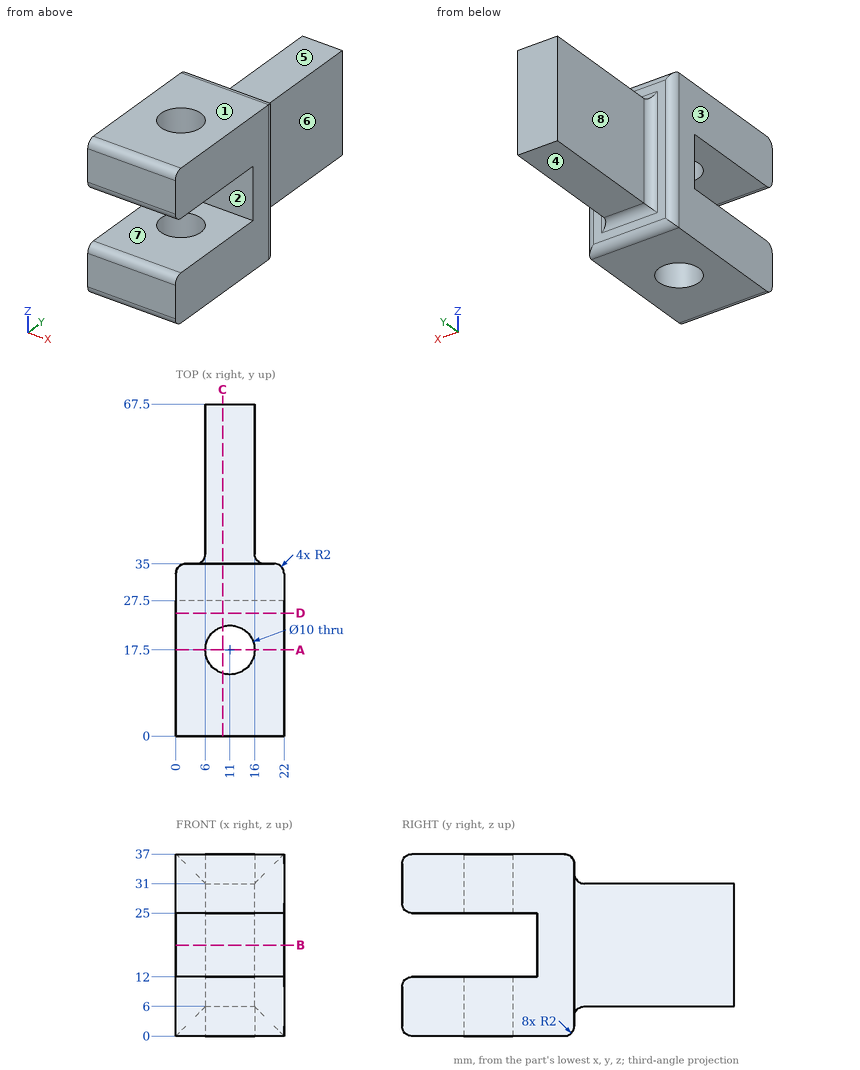
Verification items for this drawing (mm, ordinates from the low corner). A direction names the side the tool comes from. Round coordinates to 2 decimals unless told otherwise and drop trailing zeros. Order: outer loops, then holes, each group sorted by start corner. A loop starts at its lowest first (then second) coordinate and runs counter-clockwise, first axis right, second up. Notation, with made-up numbers: (34.5, 50.25) -> (88.5, 50.25) arc R11 cw to (88.5, 58.25) -> close; hole circle Ø1 at (40.5, -39). An arc over 180 degrees is marked (long way). Use one line per item in the form item = value.
1. Go/stop test with flat-tipped pins: pin 1 (5 mm diameter, centred on x = 11, y = 45.5, fed in from +Z); pin 2 (8 mm diameter, centred on y = 24.5, z = 18.5, fed in from -X); pin 3 (4 mm diameter, centred on x = 10, y = 45, fed in from -Z); pin 4 (8 mm diameter, centred on y = 56.5, z = 29, fed in from -X). Record where each tip stops, or that it passes through.
Working result:
pin_1 = 31
pin_2 = 0
pin_3 = 6
pin_4 = 6
2. Cross-section at D-D, the plane y = 25. Enter the section's corners in (x, z).
Working result:
outline = (0, 0) -> (22, 0) -> (22, 12) -> (0, 12) -> close; (0, 25) -> (22, 25) -> (22, 37) -> (0, 37) -> close
3. Cross-section at A-A, the plane y = 17.5. Enter the section's corners in (x, z).
Working result:
outline = (0, 0) -> (6, 0) -> (6, 12) -> (0, 12) -> close; (0, 25) -> (6, 25) -> (6, 37) -> (0, 37) -> close; (16, 0) -> (22, 0) -> (22, 12) -> (16, 12) -> close; (16, 25) -> (22, 25) -> (22, 37) -> (16, 37) -> close
4. Mould release check, pull along Z, two halves, no side actions. Record for the marked faces 1, 2 and 3: pulls with the +Z half, pulls with the -Z half, needs draft (parallel to the pull), parting line crosses it, or undercut.
Working result:
face_1 = pulls with the +Z half
face_2 = undercut
face_3 = needs draft
5. Scan lines: line 1 along Y through (x, z) = (11, 7.25); line 2 along Z through (x, y) = (16.75, 12); line 3 along Y through (x, z) = (11, 34.25). Record each from-to range of solid material in increasing order. Write a range as from..to.
Working result:
line_1 = 0..12.5, 22.5..67.5
line_2 = 0..12, 25..37
line_3 = 0..12.5, 22.5..35
6. Set-up check for the marked faces 4, 5, 6, 7 and 8: record each of +Z, -Z, +X, -X, +Y, -Y from which the full face is reachable in a straight line by a thin tool's end or side.
Working result:
face_4 = -Z, +X, -X, +Y
face_5 = +Z, +X, -X, +Y
face_6 = +Z, -Z, +X, +Y
face_7 = +X, -X, -Y
face_8 = +Z, -Z, -X, +Y
7. Cross-section at B-B, the plane z = 18.5. Enter the section's corners in (x, y), plus the area to 3 significant figures.
Working result:
outline = (0, 27.5) -> (22, 27.5) -> (22, 33) arc R2 ccw to (20, 35) -> (18, 35) arc R2 cw to (16, 37) -> (16, 67.5) -> (6, 67.5) -> (6, 37) arc R2 cw to (4, 35) -> (2, 35) arc R2 ccw to (0, 33) -> close
area = 490 mm^2
8. Cross-section at C-C, the plane x = 9.5. Enter the section's corners in (y, z).
Working result:
outline = (0, 2) arc R2 ccw to (2, 0) -> (12.73, 0) -> (12.73, 12) -> (2, 12) arc R2 ccw to (0, 10) -> close; (0, 27) arc R2 ccw to (2, 25) -> (12.73, 25) -> (12.73, 37) -> (2, 37) arc R2 ccw to (0, 35) -> close; (22.27, 0) -> (33, 0) arc R2 ccw to (35, 2) -> (35, 4) arc R2 cw to (37, 6) -> (67.5, 6) -> (67.5, 31) -> (37, 31) arc R2 cw to (35, 33) -> (35, 35) arc R2 ccw to (33, 37) -> (22.27, 37) -> (22.27, 25) -> (27.5, 25) -> (27.5, 12) -> (22.27, 12) -> close
